```python
from build123d import *

# Parameters (mm, degrees)
BOSS_EXTRUDE1_DEPTH = 50.8
SKETCH2_R           = 26.19375
CUT_EXTRUDE1_DEPTH  = 128
SKETCH3_R           = 3.175
CUT_EXTRUDE2_DEPTH  = 128
CIRPATTERN1_COUNT   = 5


with BuildPart() as part:
    # Sketch1 → Boss-Extrude1 (new body, symmetric)
    with BuildSketch(Plane(origin=(0, 0, 0), x_dir=(1, 0, 0), z_dir=(0, 1, 0))):
        Polygon((0, 63.5), (6.35, 63.5), (6.35, -57.15), (127, -57.15), (127, -63.5), (0, -63.5), align=None)
    extrude(amount=BOSS_EXTRUDE1_DEPTH, both=True)

    # Sketch2 → Cut-Extrude1 (cut, through all)
    with BuildSketch(Plane.ZY):
        Circle(SKETCH2_R)
    extrude(amount=-CUT_EXTRUDE1_DEPTH, mode=Mode.SUBTRACT)

    # Sketch3 → Cut-Extrude2 (cut, through all)
    with BuildSketch(Plane.ZY):
        with Locations((0, 38.89375)):
            Circle(SKETCH3_R)
    cut_extrude2 = extrude(amount=-CUT_EXTRUDE2_DEPTH, mode=Mode.SUBTRACT)

    # CirPattern1: Cut-Extrude2 ×5 about axis
    cirpattern1_axis = Axis((0, 0, 0), (1, 0, 0))
    for i in range(1, CIRPATTERN1_COUNT):
        add(cut_extrude2.rotate(cirpattern1_axis, i * 360 / CIRPATTERN1_COUNT), mode=Mode.SUBTRACT)


solid = part.part
```
Geometry check sheet. Reference: the model listing, model coordinates, mm. A direction names the side the tool comes from. Coordinates: 2 decimals unless noted, no trailing zeros. Order: outer loops, then holes, each group sorted by start corner. A loop starts at its lowest first (then second) coordinate and runs counter-clockwise, first axis right, second up.
Item 1: Depth check by flat-ended pin: pin 1 (10 mm diameter, centred on y = -31.47, z = 22.86, fed in from +X); pin 2 (5.5 mm diameter, centred on y = -31.47, z = -22.86, fed in from +X); pin 3 (3 mm diameter, centred on x = 76.5, y = 18, fed in from -Z). Enter the tip coordinate at first touch or a pass-through.
Item 2: Section check A-A (z = 0). Enter the section's corners in (x, y).
Item 3: Tool access check on faces 1 (the cylindrical face through (3.131, -30.457, -25.872)), 2 (the flat face through (6.35, 1, -31)). Record the directions out of +Z, -Z, +X, -X, +Y, -Y that give a thin tool (end or side, any length) a straight path to the whole face; none if there is none.
Item 4: Scan lines: line 1 along Y through (x, z) = (4, 0); line 2 along Z through (x, y) = (22, 43); line 3 along X through (y, z) = (-40, 17). Record each from-to range of solid material in increasing order.
Item 5: Section check D-D (y = 19). Enter the section's corners in (x, z).
Item 6: Mould release check, pull along Y, two halves, no side actions. Record for faces 3 (the flat face through (3, 50.8, 28)), 4 (the cylindrical face through (3.13, -28.42, 23.76)), 5 (the flat face through (0, 23, 15)), 6 (the cylindrical face through (3.131, 42.042, -0.413)): released by +Y, released by -Y, zero draft, split by the parting line, or undercut.
Item 7: Section check C-C (z = -13.5). Enter the section's corners in (x, y).
Item 8: Section check B-B (y = 0). Enter the section's corners in (x, z).
Check sheet entries:
1. pin 1: stops at x = 6.35
1. pin 2: passes through
1. pin 3: stops at z = 57.15
2. outline: (0, -50.8) - (6.35, -50.8) - (6.35, -26.19) - (0, -26.19) - close; (0, 26.19) - (6.35, 26.19) - (6.35, 35.72) - (0, 35.72) - close; (0, 42.07) - (6.35, 42.07) - (6.35, 50.8) - (0, 50.8) - close
3. face 1: +X, -X
3. face 2: -Z, +X, +Y, -Y
4. line 1: y = -50.8 to -26.19, 26.19 to 35.72, 42.07 to 50.8
4. line 2: z = 57.15 to 63.5
4. line 3: x = 0 to 6.35
5. outline: (0, -63.5) - (6.35, -63.5) - (6.35, -18.03) - (0, -18.03) - close; (0, 18.03) - (6.35, 18.03) - (6.35, 57.15) - (127, 57.15) - (127, 63.5) - (0, 63.5) - close
6. face 3: released by +Y
6. face 4: undercut
6. face 5: zero draft
6. face 6: undercut
7. outline: (0, -50.8) - (6.35, -50.8) - (6.35, -22.45) - (0, -22.45) - close; (0, 22.45) - (6.35, 22.45) - (6.35, 50.8) - (0, 50.8) - close
8. outline: (0, -63.5) - (6.35, -63.5) - (6.35, -26.19) - (0, -26.19) - close; (0, 26.19) - (6.35, 26.19) - (6.35, 57.15) - (127, 57.15) - (127, 63.5) - (0, 63.5) - close
